Geometry check sheet. Reference: the model listing, model coordinates, mm. Face numbers are marked on the shaded views. A direction names the side the tool comes from. Give positions to 0.01 mm unless a question says otherwise; leave off trailing zeros. Loops run counter-clockwise (first coordinate to the right, second up) from the corner with the lowest first, then second, coordinate; pieces in that order, holes last. Notation, with made-up numbers: (74, 86) -> (91, 86) arc R17 cw to (91, 100) -> close; hole circle Ø1 at (39, 25). An arc over 180 degrees is marked (long way). One line per item, written item: value. Start each with the question number.
(1) Draft check along Z on the marked faces 1 and 2. Enter one of: pulls with the +Z half, pulls with the -Z half, needs draft (parallel to the pull), parting line crosses it, or undercut.
(2) Gauge pin test, flat ends, axial feed: pin 1 Ø0.8 at (x, z) = (37, -1.5) entering from -Y; pin 2 Ø1.3 at (y, z) = (89.5, 26.5) entering from +X; pin 3 Ø0.8 at (x, z) = (106.5, 27.5) entering from -Y; pin 4 Ø1 at (x, z) = (104, 24) entering from -Y. Record the tip position at first contact, or that the pin passes through.
(3) Sectioned sample at D-D, the plane y = 18.5. Record the cut outline in (x, z), then the cut area to 3 significant figures.
(4) Tool access check on the marked faces 3, 4, 5 and 6. Record the directions out of +Z, -Z, +X, -X, +Y, -Y that give a thin tool (end or side, any length) a straight path to the whole face; none if there is none.
(5) Sectioned sample at A-A, the plane y = -69. Record the cut outline in (x, z), then the cut area to 3 significant figures.
(6) Scan lines: line 1 along X through (y, z) = (0, -1) (3 decimals); line 2 along Z through (x, y) = (34, -18.5). Record each from-to range of solid material in increasing order. Write a range as from..to.
(7) Sectioned sample at B-B, the plane x = -35. Record the cut outline in (y, z).
(8) Sectioned sample at C-C, the plane z = 5.5. Record the cut outline in (x, y), then the cut area to 3 significant figures.
from build123d import *

# Parameters (mm, degrees)
F0_R     = 41.91
F1_DEPTH = 25.4
F2_W     = 25.4
F2_H     = 139.7
F2_W_2   = 139.7
F2_H_2   = 25.4
F3_DEPTH = 2.54
F4_W     = 9.525
F4_H     = 43.4975
F4_W_2   = 43.4975
F4_H_2   = 9.525
F4_R     = 3.175
F5_DEPTH = 2.54


with BuildPart() as f1:
    # F0 (on Top) → F1 (new body)
    with BuildSketch(Plane.XY):
        Circle(F0_R)
    extrude(amount=F1_DEPTH)

    # F2 (on face) → F3 (join)
    with BuildSketch(Plane.XY.offset(25.4)):
        with Locations((0, 82.55)):
            Rectangle(F2_W, F2_H)
        with Locations((82.55, 0)):
            Rectangle(F2_W_2, F2_H_2)
        Rectangle(F2_W, F2_H_2)
        with Locations((-82.55, 0)):
            Rectangle(F2_W_2, F2_H_2)
        with Locations((0, -82.55)):
            Rectangle(F2_W, F2_H)
    extrude(amount=F3_DEPTH)

    # F4 (on face) → F5 (join)
    with BuildSketch(Plane(origin=(0, 0, 0), x_dir=(1, 0, 0), z_dir=(0, 0, -1))):
        with Locations((0, -26.51125)):
            Rectangle(F4_W, F4_H)
        with Locations((-26.51125, 0)):
            Rectangle(F4_W_2, F4_H_2)
        Rectangle(F4_W, F4_H_2)
        Circle(F4_R, mode=Mode.SUBTRACT)
        with Locations((26.51125, 0)):
            Rectangle(F4_W_2, F4_H_2)
        with Locations((0, 26.51125)):
            Rectangle(F4_W, F4_H)
    extrude(amount=F5_DEPTH)


solid = f1.part
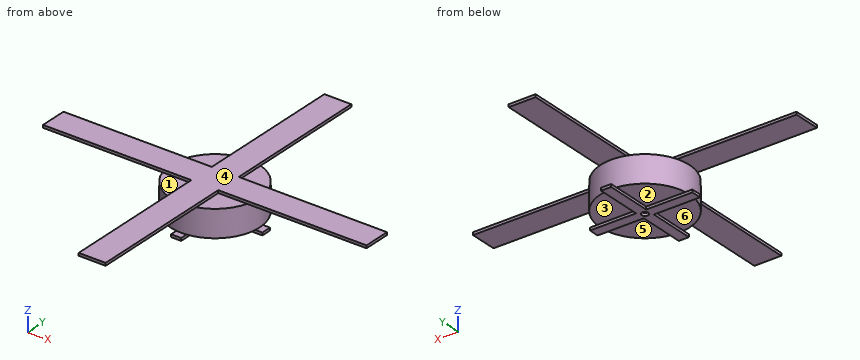
Calculated:
1. face 1: pulls with the +Z half
1. face 2: pulls with the -Z half
2. pin 1: stops at y = -4.76
2. pin 2: stops at x = 12.7
2. pin 3: stops at y = -12.7
2. pin 4: passes through
3. outline: (-37.61, 0) -> (-4.76, 0) -> (-4.76, -2.54) -> (4.76, -2.54) -> (4.76, 0) -> (37.61, 0) -> (37.61, 25.4) -> (12.7, 25.4) -> (12.7, 27.94) -> (-12.7, 27.94) -> (-12.7, 25.4) -> (-37.61, 25.4) -> close
3. area: 2,000 mm2
4. face 3: -Z, +X, +Y
4. face 4: +Z, +X, -X, +Y, -Y
4. face 5: -Z, +X, -Y
4. face 6: -Z, -X, -Y
5. outline: (-12.7, 25.4) -> (12.7, 25.4) -> (12.7, 27.94) -> (-12.7, 27.94) -> close
5. area: 64.5 mm2
6. line 1: x = -48.26..-3.175, 3.175..48.26
6. line 2: z = 0..25.4
7. outline: (-23.05, 0) -> (-4.76, 0) -> (-4.76, -2.54) -> (4.76, -2.54) -> (4.76, 0) -> (23.05, 0) -> (23.05, 25.4) -> (12.7, 25.4) -> (12.7, 27.94) -> (-12.7, 27.94) -> (-12.7, 25.4) -> (-23.05, 25.4) -> close
8. outline: circle Ø83.82 at (0, 0)
8. area: 5,520 mm2
